from build123d import *

# Parameters (mm, degrees)
BOSS_EXTRUDE1_DEPTH = 101.6
CHAMFER1_SIZE       = 6
CHAMFER1_SIZE2      = 5.57330498
FILLET1_R           = 4
SKETCH2_W           = 6
SKETCH2_H           = 20
BOSS_EXTRUDE2_DEPTH = 5


with BuildPart() as part:
    # Sketch1 → Boss-Extrude1 (new body)
    with BuildSketch(Plane.XY):
        Polygon((-33.412698413, -41.573204241), (16.587301587, -37.573204241), (16.587301587, -34.573204241), (-23.412698413, -34.573204241), (-23.412698413, 18.426795759), (-33.412698413, 18.426795759), (-33.412698413, -33.573204241), align=None)
    extrude(amount=BOSS_EXTRUDE1_DEPTH)

    # Chamfer1
    chamfer1_edges = [part.edges().sort_by_distance(p)[0] for p in [
        (-33.412698413, -41.573204241, 50.8),
    ]]
    chamfer1_side = [part.faces().sort_by_distance(p)[0] for p in [
        (-33.412698413, -11.573204241, 50.8),
    ]]
    chamfer(chamfer1_edges, length=CHAMFER1_SIZE, length2=CHAMFER1_SIZE2, reference=chamfer1_side[0])

    # Fillet1
    fillet1_edges = [part.edges().sort_by_distance(p)[0] for p in [
        (-23.412698413, -34.573204241, 50.8),
    ]]
    fillet(fillet1_edges, radius=FILLET1_R)

    # Sketch2 → Boss-Extrude2 (add)
    with BuildSketch(Plane(origin=(0, 18.426795759, 0), x_dir=(1, 0, 0), z_dir=(0, 1, 0))):
        with Locations((-30.412698413, -91.6)):
            Rectangle(SKETCH2_W, SKETCH2_H)
        with Locations((-30.412698413, -10)):
            Rectangle(SKETCH2_W, SKETCH2_H)
    extrude(amount=BOSS_EXTRUDE2_DEPTH)


solid = part.part
The listing builds one solid part. Answer for the finished solid, in the listing's coordinates (mm). A direction names the side the tool comes from. Give positions to 0.01 mm unless a question says otherwise; leave off trailing zeros. Write each loop counter-clockwise with the first axis right and the second up, starting at its lowest first coordinate (ties: lowest second). Pieces come first, ordered by that corner, then holes.
1) Find the intervals of material crossed by L1, parallel to X at y = -30, z = 14; L2, parallel to Y at x = -21.5, z = 45.5; L3, parallel to Y at x = 12, z = 9, in increasing order.
2) Section D-D (z = 77) is taken. Write down the section's boundary in (x, y).
3) Section B-B (y = -15) is taken. Write down the section's boundary in (x, z), and give its area (3 significant figures).
4) A tool of negligible diameter and unlimited length cuts with its end or side. For faces 4 (the face through (-30, 23.427, 91)), 5 (the face through (-27.413, 21, 92)), 6 (the face through (-30, 21, 81.6)), from which of +Z, -Z, +X, -X, +Y, -Y can it reach the whole face along a straight path? Write none if from no direction.
5) Given P1, Ø6, axis at y = 13.5, z = 29.5, coming from the +X side; P2, Ø3, axis at x = -21.5, z = 27.5, coming from the -Y side; P3, Ø12, axis at x = -4, z = 81.5, coming from the -Y side, each flat-ended and moving along its own axis, determine where each tip first touches the part or whether it passes through.
6) Section A-A (z = 17) is taken. Write down the section's boundary in (x, y), and give its area (3 significant figures).
7) Section C-C (x = 12) is taken. Write down the section's boundary in (y, z).
8) For a pull along Z with two mould halves and no side action, classify faces 1 (the face through (-30, 21, 20)), 2 (the face through (16.587, -36, 50)), 3 (the face through (-25, -18, 0)) as pulls with the +Z half, pulls with the -Z half, needs draft (parallel to the pull), parting line crosses it, or undercut.
Response:
1. L1: x = -33.41 to -23.41
1. L2: y = -40.62 to -33.99
1. L3: y = -37.94 to -34.57
2. outline: (-33.41, -35.57) - (-27.86, -41.13) - (16.59, -37.57) - (16.59, -34.57) - (-19.41, -34.57) arc R4 cw to (-23.41, -30.57) - (-23.41, 18.43) - (-33.41, 18.43) - close
3. outline: (-33.41, 0) - (-23.41, 0) - (-23.41, 101.6) - (-33.41, 101.6) - close
3. area: 1,020 mm2
4. face 4: +Z, -Z, +X, -X, +Y
4. face 5: +Z, -Z, +X, +Y
4. face 6: +X, -X, +Y
5. P1: stops at x = -23.41
5. P2: stops at y = -40.74
5. P3: stops at y = -39.7
6. outline: (-33.41, -35.57) - (-27.86, -41.13) - (16.59, -37.57) - (16.59, -34.57) - (-19.41, -34.57) arc R4 cw to (-23.41, -30.57) - (-23.41, 18.43) - (-27.41, 18.43) - (-27.41, 23.43) - (-33.41, 23.43) - close
6. area: 797 mm2
7. outline: (-37.94, 0) - (-34.57, 0) - (-34.57, 101.6) - (-37.94, 101.6) - close
8. face 1: undercut
8. face 2: needs draft
8. face 3: pulls with the -Z half
